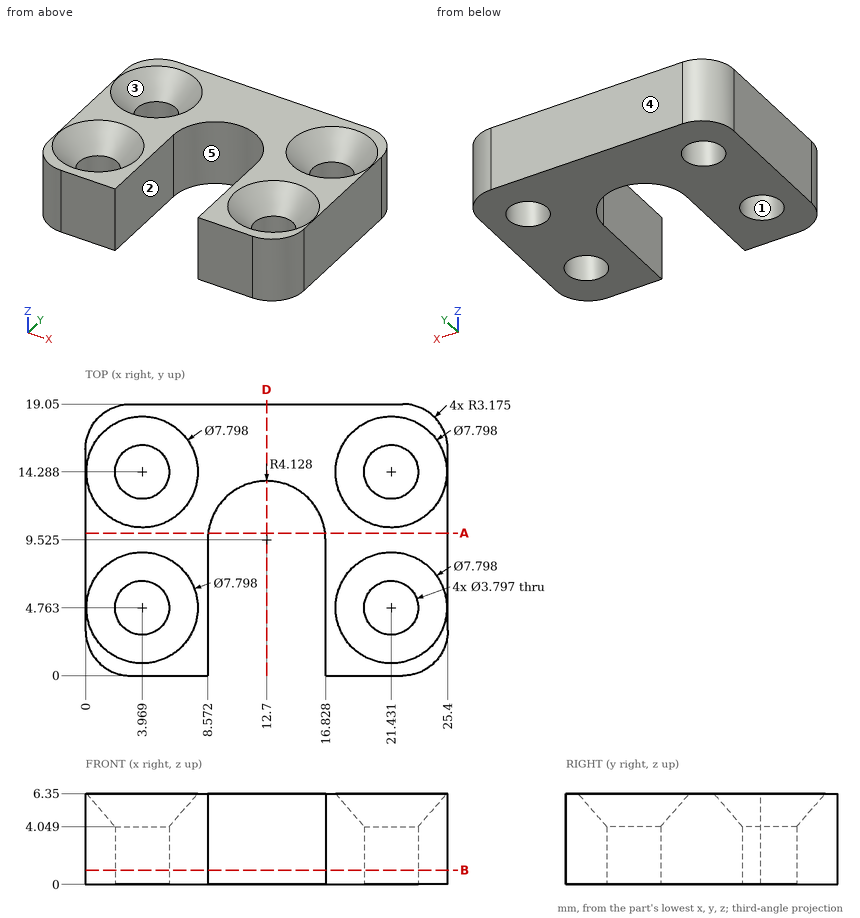
Geometry check sheet. Reference: drawing and pictorial views, mm from the part's lowest x, y, z. A direction names the side the tool comes from. Round coordinates to 2 decimals unless told otherwise and drop trailing zeros. Loops run counter-clockwise (first coordinate to the right, second up) from the corner with the lowest first, then second, coordinate; pieces in that order, holes last. Notation, with made-up numbers: (49.25, 29) - (94.25, 29) arc R30 cw to (94.25, 52) - close; hole circle Ø3 at (49.25, -6). An arc over 180 degrees is marked (long way). Write item = value, one per line. Start each with the question number.
Q1. Section check A-A (y = 10). Record the boundary of the cut face in (x, z), plus the area to 3 significant figures.
Q2. Access from +Z, -Z, +X, -X, +Y, -Y to the whole of each face (thin tool, end or side, straight path). Record for the marked faces 1 and 2.
Q3. Depth check by flat-ended pin: P1, Ø6, axis at x = 21.43, y = 4.76, coming from the +Z side. Enter the tip coordinate at first touch or a pass-through.
Q4. Thickness scan on L1, parallel to X at y = 9, z = 6.25; L2, parallel to X at y = 15, z = 2; L3, parallel to Y at x = 22.5, z = 4.75 (1 decimal). Record the ranges inside material, lowest first.
Q5. Section check D-D (x = 12.7). Record the boundary of the cut face in (y, z).
Q6. Section check B-B (z = 1). Count the separate pieces of the cut face and the enclosed holes in it.
Q7. Release check for a two-part mould opening along Y. For the marked faces 3, 4 and 5 record: pulls with the +Y half, pulls with the -Y half, needs draft (parallel to the pull), parting line crosses it, or undercut.
Derived:
q1.outline = (0, 0) - (8.6, 0) - (8.6, 6.35) - (0, 6.35) - close; (16.8, 0) - (25.4, 0) - (25.4, 6.35) - (16.8, 6.35) - close
q1.area = 109 mm^2
q2.face_1 = +Z, -Z
q2.face_2 = +Z, -Z, -Y
q3.P1 = 5.32
q4.L1 = 0 to 8.57, 16.83 to 25.4
q4.L2 = 0 to 2.21, 5.73 to 19.67, 23.19 to 25.4
q4.L3 = 0 to 2.5, 7 to 12, 16.6 to 19
q5.outline = (13.65, 0) - (19.05, 0) - (19.05, 6.35) - (13.65, 6.35) - close
q6.separate_pieces = 1
q6.enclosed_holes = 4
q7.face_3 = undercut
q7.face_4 = pulls with the +Y half
q7.face_5 = pulls with the -Y half
